```python
from build123d import *

# Parameters (mm, degrees)
SALIENTE_EXTRUIR1_DEPTH = 30


with BuildPart() as part:
    # Croquis1 → Saliente-Extruir1 (new body)
    with BuildSketch(Plane.XY):
        with BuildLine():
            Line((-8, 0), (-5, 0))
            ThreePointArc((-5, 0), (0, 5), (5, 0))
            Line((5, 0), (8, 0))
            ThreePointArc((8, 0), (6.891439137, 4.063012013), (3.872983346, 7))
            Line((3.872983346, 7), (-3.872983346, 7))
            ThreePointArc((-3.872983346, 7), (-6.891439137, 4.063012013), (-8, 0))
        make_face()
    extrude(amount=SALIENTE_EXTRUIR1_DEPTH)


solid = part.part
```
Input: part model. Units: mm. Frame: model coordinates. Give positions to 0.01 mm unless a question says otherwise; leave off trailing zeros. Write each loop counter-clockwise with the first axis right and the second up, starting at its lowest first coordinate (ties: lowest second). Pieces come first, ordered by that corner, then holes. Notation, with made-up numbers: (-25, -16.75) - (14, -16.75) arc R29 cw to (14, 12.25) - close; hole circle Ø11 at (65.25, 48). An arc over 180 degrees is marked (long way). Write item = value, one per line. Start each with the question number.
1. Section query D-D, the plane x = 0. Output: boundary loops of the cut face in (y, z).
2. Ray query, L1, parallel to X at y = 0.5, z = 19; L2, parallel to X at y = 2.75, z = 22; L3, parallel to Y at x = 1.25, z = 14.5. Return the intervals inside material, ascending.
3. Section query B-B, the plane z = 15.5. Output: boundary loops of the cut face in (x, y).
4. Section query C-C, the plane y = 2. Output: boundary loops of the cut face in (x, z), then the cut area to 3 significant figures.
5. First-contact query: pin 1 Ø6 at (x, z) = (1.5, 5.5) entering from -Y; pin 2 Ø3 at (y, z) = (2, 5) entering from +X. Flat tips, straight axial feed; report the tip coordinate or a pass-through.
6. Section query A-A, the plane y = 3.75. Output: boundary loops of the cut face in (x, z), then the cut area to 3 significant figures.
Check sheet entries:
q1.outline = (5, 0) - (7, 0) - (7, 30) - (5, 30) - close
q2.L1 = -7.98 to -4.97, 4.97 to 7.98
q2.L2 = -7.51 to -4.18, 4.18 to 7.51
q2.L3 = 4.84 to 7
q3.outline = (-8, 0) - (-5, 0) arc R5 cw to (5, 0) - (8, 0) arc R8 ccw to (3.87, 7) - (-3.87, 7) arc R8 ccw to start
q4.outline = (-7.75, 0) - (-4.58, 0) - (-4.58, 30) - (-7.75, 30) - close; (4.58, 0) - (7.75, 0) - (7.75, 30) - (4.58, 30) - close
q4.area = 190 mm2
q5.pin_1 = 2.18
q5.pin_2 = 7.98
q6.outline = (-7.07, 0) - (-3.31, 0) - (-3.31, 30) - (-7.07, 30) - close; (3.31, 0) - (7.07, 0) - (7.07, 30) - (3.31, 30) - close
q6.area = 226 mm2
